```python
from build123d import *

# Parameters (mm, degrees)
BOSS_EXTRUDE1_DEPTH = 10
CUT_EXTRUDE5_REACH  = 12
SKETCH8_R           = 2.6
SKETCH9_R           = 4.1
CUT_EXTRUDE6_DEPTH  = 5.4
CUT_EXTRUDE7_REACH  = 89
SKETCH11_R          = 1.6
CUT_EXTRUDE8_DEPTH  = 3
CUT_EXTRUDE9_REACH  = 12
SKETCH14_R          = 1.55
CUT_EXTRUDE10_DEPTH = 2.6


with BuildPart() as part:
    # Sketch1 → Boss-Extrude1 (new body)
    with BuildSketch(Plane(origin=(0, 0, 0), x_dir=(1, 0, 0), z_dir=(0, 1, 0))):
        with BuildLine():
            Line((0, 11), (0, 51))
            ThreePointArc((0, 51), (3.221825407, 58.778174593), (11, 62))
            Line((11, 62), (76, 62))
            ThreePointArc((76, 62), (83.778174593, 58.778174593), (87, 51))
            Line((87, 51), (87, 11))
            ThreePointArc((87, 11), (83.778174593, 3.221825407), (76, 0))
            Line((76, 0), (11, 0))
            ThreePointArc((11, 0), (3.221825407, 3.221825407), (0, 11))
        make_face()
    extrude(amount=BOSS_EXTRUDE1_DEPTH)

    # Sketch8 → Cut-Extrude5 (cut, up to next)
    with BuildSketch(Plane(origin=(0, 10, 0), x_dir=(1, 0, 0), z_dir=(0, 1, 0)), mode=Mode.PRIVATE) as cut_extrude5_sk1:
        with Locations((75.7, 51)):
            Circle(SKETCH8_R)
    cut_extrude5_tool1 = extrude(cut_extrude5_sk1.sketch, amount=-CUT_EXTRUDE5_REACH, mode=Mode.PRIVATE) & part.part
    add(cut_extrude5_tool1.solids().sort_by_distance((75.7, 10, -51))[0], mode=Mode.SUBTRACT)
    # Sketch8 → Cut-Extrude5 (cut, up to next)
    with BuildSketch(Plane(origin=(0, 10, 0), x_dir=(1, 0, 0), z_dir=(0, 1, 0)), mode=Mode.PRIVATE) as cut_extrude5_sk2:
        with Locations((75.7, 11)):
            Circle(SKETCH8_R)
    cut_extrude5_tool2 = extrude(cut_extrude5_sk2.sketch, amount=-CUT_EXTRUDE5_REACH, mode=Mode.PRIVATE) & part.part
    add(cut_extrude5_tool2.solids().sort_by_distance((75.7, 10, -11))[0], mode=Mode.SUBTRACT)
    # Sketch8 → Cut-Extrude5 (cut, up to next)
    with BuildSketch(Plane(origin=(0, 10, 0), x_dir=(1, 0, 0), z_dir=(0, 1, 0)), mode=Mode.PRIVATE) as cut_extrude5_sk3:
        with BuildLine():
            Line((10, 53.6), (21, 53.6))
            ThreePointArc((21, 53.6), (23.6, 51), (21, 48.4))
            Line((21, 48.4), (10, 48.4))
            ThreePointArc((10, 48.4), (7.4, 51), (10, 53.6))
        make_face()
    cut_extrude5_tool3 = extrude(cut_extrude5_sk3.sketch, amount=-CUT_EXTRUDE5_REACH, mode=Mode.PRIVATE) & part.part
    add(cut_extrude5_tool3.solids().sort_by_distance((15.5, 10, -51))[0], mode=Mode.SUBTRACT)
    # Sketch8 → Cut-Extrude5 (cut, up to next)
    with BuildSketch(Plane(origin=(0, 10, 0), x_dir=(1, 0, 0), z_dir=(0, 1, 0)), mode=Mode.PRIVATE) as cut_extrude5_sk4:
        with BuildLine():
            Line((10, 13.6), (21, 13.6))
            ThreePointArc((21, 13.6), (23.6, 11), (21, 8.4))
            Line((21, 8.4), (10, 8.4))
            ThreePointArc((10, 8.4), (7.4, 11), (10, 13.6))
        make_face()
    cut_extrude5_tool4 = extrude(cut_extrude5_sk4.sketch, amount=-CUT_EXTRUDE5_REACH, mode=Mode.PRIVATE) & part.part
    add(cut_extrude5_tool4.solids().sort_by_distance((15.5, 10, -11))[0], mode=Mode.SUBTRACT)

    # Sketch9 → Cut-Extrude6 (cut)
    with BuildSketch(Plane.XZ):
        with Locations((75.7, -11)):
            Circle(SKETCH9_R)
        with Locations((75.7, -51)):
            Circle(SKETCH9_R)
        with BuildLine():
            Line((10, -6.9), (21, -6.9))
            ThreePointArc((21, -6.9), (25.1, -11), (21, -15.1))
            Line((21, -15.1), (10, -15.1))
            ThreePointArc((10, -15.1), (8.336419524, -14.747332385), (6.95902976, -13.75))
            Line((6.95902976, -13.75), (3, -13.75))
            Line((3, -13.75), (3, -8.25))
            Line((3, -8.25), (6.95902976, -8.25))
            ThreePointArc((6.95902976, -8.25), (8.336419524, -7.252667615), (10, -6.9))
        make_face()
        with BuildLine():
            Line((10, -46.9), (21, -46.9))
            ThreePointArc((21, -46.9), (25.1, -51), (21, -55.1))
            Line((21, -55.1), (10, -55.1))
            ThreePointArc((10, -55.1), (8.336419524, -54.747332385), (6.95902976, -53.75))
            Line((6.95902976, -53.75), (3, -53.75))
            Line((3, -53.75), (3, -48.25))
            Line((3, -48.25), (6.95902976, -48.25))
            ThreePointArc((6.95902976, -48.25), (8.336419524, -47.252667615), (10, -46.9))
        make_face()
    extrude(amount=-CUT_EXTRUDE6_DEPTH, mode=Mode.SUBTRACT)

    # Sketch11 → Cut-Extrude7 (cut, up to next)
    with BuildSketch(Plane.ZY, mode=Mode.PRIVATE) as cut_extrude7_sk1:
        with Locations((-11, 5)):
            Circle(SKETCH11_R)
    cut_extrude7_tool1 = extrude(cut_extrude7_sk1.sketch, amount=-CUT_EXTRUDE7_REACH, mode=Mode.PRIVATE) & part.part
    add(cut_extrude7_tool1.solids().sort_by_distance((0, 5, -11))[0], mode=Mode.SUBTRACT)
    # Sketch11 → Cut-Extrude7 (cut, up to next)
    with BuildSketch(Plane.ZY, mode=Mode.PRIVATE) as cut_extrude7_sk2:
        with Locations((-51, 5)):
            Circle(SKETCH11_R)
    cut_extrude7_tool2 = extrude(cut_extrude7_sk2.sketch, amount=-CUT_EXTRUDE7_REACH, mode=Mode.PRIVATE) & part.part
    add(cut_extrude7_tool2.solids().sort_by_distance((0, 5, -51))[0], mode=Mode.SUBTRACT)

    # Sketch12 → Cut-Extrude8 (cut)
    with BuildSketch(Plane(origin=(3, 0, 0), x_dir=(0, 0, -1), z_dir=(1, 0, 0))):
        Polygon((48.25, 6.58771324), (48.25, 3.41228676), (51, 1.824573519), (53.75, 3.41228676), (53.75, 6.58771324), (51, 8.175426481), align=None)
        Polygon((13.75, 3.41228676), (13.75, 6.58771324), (11, 8.175426481), (8.25, 6.58771324), (8.25, 3.41228676), (11, 1.824573519), align=None)
    extrude(amount=CUT_EXTRUDE8_DEPTH, mode=Mode.SUBTRACT)

    # Sketch14 → Cut-Extrude9 (cut, up to next)
    with BuildSketch(Plane(origin=(0, 10, 0), x_dir=(1, 0, 0), z_dir=(0, 1, 0)), mode=Mode.PRIVATE) as cut_extrude9_sk1:
        with Locations((30.5, 47)):
            Circle(SKETCH14_R)
    cut_extrude9_tool1 = extrude(cut_extrude9_sk1.sketch, amount=-CUT_EXTRUDE9_REACH, mode=Mode.PRIVATE) & part.part
    add(cut_extrude9_tool1.solids().sort_by_distance((30.5, 10, -47))[0], mode=Mode.SUBTRACT)
    # Sketch14 → Cut-Extrude9 (cut, up to next)
    with BuildSketch(Plane(origin=(0, 10, 0), x_dir=(1, 0, 0), z_dir=(0, 1, 0)), mode=Mode.PRIVATE) as cut_extrude9_sk2:
        with Locations((56.5, 47)):
            Circle(SKETCH14_R)
    cut_extrude9_tool2 = extrude(cut_extrude9_sk2.sketch, amount=-CUT_EXTRUDE9_REACH, mode=Mode.PRIVATE) & part.part
    add(cut_extrude9_tool2.solids().sort_by_distance((56.5, 10, -47))[0], mode=Mode.SUBTRACT)
    # Sketch14 → Cut-Extrude9 (cut, up to next)
    with BuildSketch(Plane(origin=(0, 10, 0), x_dir=(1, 0, 0), z_dir=(0, 1, 0)), mode=Mode.PRIVATE) as cut_extrude9_sk3:
        with Locations((30.5, 15)):
            Circle(SKETCH14_R)
    cut_extrude9_tool3 = extrude(cut_extrude9_sk3.sketch, amount=-CUT_EXTRUDE9_REACH, mode=Mode.PRIVATE) & part.part
    add(cut_extrude9_tool3.solids().sort_by_distance((30.5, 10, -15))[0], mode=Mode.SUBTRACT)
    # Sketch14 → Cut-Extrude9 (cut, up to next)
    with BuildSketch(Plane(origin=(0, 10, 0), x_dir=(1, 0, 0), z_dir=(0, 1, 0)), mode=Mode.PRIVATE) as cut_extrude9_sk4:
        with Locations((56.5, 15)):
            Circle(SKETCH14_R)
    cut_extrude9_tool4 = extrude(cut_extrude9_sk4.sketch, amount=-CUT_EXTRUDE9_REACH, mode=Mode.PRIVATE) & part.part
    add(cut_extrude9_tool4.solids().sort_by_distance((56.5, 10, -15))[0], mode=Mode.SUBTRACT)

    # Sketch15 → Cut-Extrude10 (cut)
    with BuildSketch(Plane.XZ):
        Polygon((33.733161507, -15), (32.116580754, -12.2), (28.883419246, -12.2), (27.266838493, -15), (28.883419246, -17.8), (32.116580754, -17.8), align=None)
        Polygon((59.733161507, -15), (58.116580754, -12.2), (54.883419246, -12.2), (53.266838493, -15), (54.883419246, -17.8), (58.116580754, -17.8), align=None)
        Polygon((59.733161507, -47), (58.116580754, -44.2), (54.883419246, -44.2), (53.266838493, -47), (54.883419246, -49.8), (58.116580754, -49.8), align=None)
        Polygon((33.733161507, -47), (32.116580754, -44.2), (28.883419246, -44.2), (27.266838493, -47), (28.883419246, -49.8), (32.116580754, -49.8), align=None)
    extrude(amount=-CUT_EXTRUDE10_DEPTH, mode=Mode.SUBTRACT)


solid = part.part
```
Geometry check sheet. Reference: the model listing, model coordinates, mm. A direction names the side the tool comes from. Coordinates: 2 decimals unless noted, no trailing zeros. Loops run counter-clockwise (first coordinate to the right, second up) from the corner with the lowest first, then second, coordinate; pieces in that order, holes last. Notation, with made-up numbers: (18.25, 54) -> (51.25, 54) arc R14 cw to (51.25, 80) -> close; hole circle Ø8 at (25, -29). An arc over 180 degrees is marked (long way). Put each result on its own line as item: value.
1) Cross-section at A-A on x = 30.5. Record the boundary of the cut face in (y, z).
Result set:
outline: (0, -62) -> (10, -62) -> (10, -48.55) -> (2.6, -48.55) -> (2.6, -49.8) -> (0, -49.8) -> close; (0, -44.2) -> (2.6, -44.2) -> (2.6, -45.45) -> (10, -45.45) -> (10, -16.55) -> (2.6, -16.55) -> (2.6, -17.8) -> (0, -17.8) -> close; (0, -12.2) -> (2.6, -12.2) -> (2.6, -13.45) -> (10, -13.45) -> (10, 0) -> (0, 0) -> close
2) Tool access check on faces 1 (the cylindrical face through (6.7, 6.6, -11)), 2 (the flat face through (16, 8, -8.4)), 3 (the flat face through (5, 3, -13.75)). Record the directions out of +Z, -Z, +X, -X, +Y, -Y that give a thin tool (end or side, any length) a straight path to the whole face; none if there is none.
Result set:
face 1: -X, -Y
face 2: +Y, -Y
face 3: -Y
3) Gauge pin test, flat ends, axial feed: pin 1 Ø4.5 at (x, y) = (4, 4.5) entering from +Z; pin 2 Ø2.5 at (x, z) = (76.5, -9.5) entering from -Y. Record the tip position at first contact, or that the pin passes through.
Result set:
pin 1: stops at z = -1.08
pin 2: stops at y = 5.4
4) Cross-section at B-B on x = 20. Record the boundary of the cut face in (y, z).
Result set:
outline: (0, -62) -> (10, -62) -> (10, -53.6) -> (5.4, -53.6) -> (5.4, -55.1) -> (0, -55.1) -> close; (0, -46.9) -> (5.4, -46.9) -> (5.4, -48.4) -> (10, -48.4) -> (10, -13.6) -> (5.4, -13.6) -> (5.4, -15.1) -> (0, -15.1) -> close; (0, -6.9) -> (5.4, -6.9) -> (5.4, -8.4) -> (10, -8.4) -> (10, 0) -> (0, 0) -> close
5) Release check for a two-part mould opening along X. For faces 4 (the flat face through (30, 1, -17.8)), 5 (the flat face through (0, 5, -31)), 6 (the cylindrical face through (1.48, 5.07, -12.6)) record: released by +X, released by -X, zero draft, split by the parting line, or undercut.
Result set:
face 4: undercut
face 5: released by -X
face 6: zero draft
6) Thickness scan on line 1 (Z direction, x = 75.7, y = 3.45); line 2 (Z direction, x = 2.35, y = 5); line 3 (X direction, y = 5, z = -8). Record the ranges inside material, lowest first.
Result set:
line 1: z = -62 to -55.1, -46.9 to -15.1, -6.9 to 0
line 2: z = -57.8 to -52.6, -49.4 to -12.6, -9.4 to -4.2
line 3: x = 0.42 to 7.21, 23.79 to 72.91, 78.49 to 86.58
